Verification items for the finished model (mm, model axes). Face numbers are marked on the shaded views. Coordinates: 2 decimals unless noted, no trailing zeros. Order: outer loops, then holes, each group sorted by start corner. A loop starts at its lowest first (then second) coordinate and runs counter-clockwise, first axis right, second up. Notation, with made-up numbers: M 3,-6 L 38,-6 A19 ccw 38,7 Z; hole C -25.75,84 d6. An arc over 180 degrees is marked long. Return JSON: item names as keys, results as strings.
```python
from build123d import *

# Parameters (mm, degrees)
SKETCH1_W           = 400
SKETCH1_H           = 76.2
BOSS_EXTRUDE1_DEPTH = 50.8
SKETCH2_R           = 19
CUT_EXTRUDE1_DEPTH  = 76.2


with BuildPart() as part:
    # Sketch1 → Boss-Extrude1 (new body)
    with BuildSketch(Plane(origin=(0, 0, 0), x_dir=(1, 0, 0), z_dir=(0, 1, 0))):
        with Locations((200, 38.1)):
            Rectangle(SKETCH1_W, SKETCH1_H)
    extrude(amount=BOSS_EXTRUDE1_DEPTH)

    # Sketch2 → Cut-Extrude1 (cut)
    with BuildSketch(Plane.XY):
        with Locations((70, 25.4)):
            Circle(SKETCH2_R)
        with Locations((200, 25.4)):
            Circle(SKETCH2_R)
        with Locations((330, 25.4)):
            Circle(SKETCH2_R)
    extrude(amount=-CUT_EXTRUDE1_DEPTH, mode=Mode.SUBTRACT)


solid = part.part
```
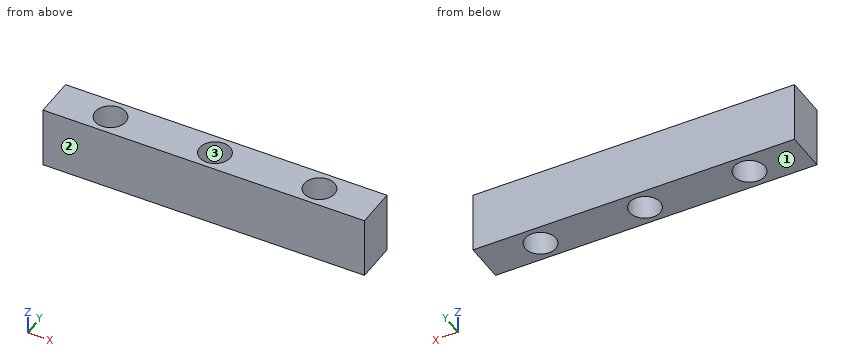
Q1. Cross-section at A-A, the plane y = 25.4. Record the boundary of the cut face in (x, z).
Values:
{"outline": "M 0,-76.2 L 51,-76.2 L 51,0 L 0,0 Z; M 89,-76.2 L 181,-76.2 L 181,0 L 89,0 Z; M 219,-76.2 L 311,-76.2 L 311,0 L 219,0 Z; M 349,-76.2 L 400,-76.2 L 400,0 L 349,0 Z"}
Q2. Cross-section at B-B, the plane x = 200. Record the boundary of the cut face in (y, z).
Values:
{"outline": "M 0,-76.2 L 6.4,-76.2 L 6.4,0 L 0,0 Z; M 44.4,-76.2 L 50.8,-76.2 L 50.8,0 L 44.4,0 Z"}
Q3. Cross-section at D-D, the plane x = 72. Record the boundary of the cut face in (y, z).
Values:
{"outline": "M 0,-76.2 L 6.51,-76.2 L 6.51,0 L 0,0 Z; M 44.29,-76.2 L 50.8,-76.2 L 50.8,0 L 44.29,0 Z"}
Q4. Go/stop test with a flat-tipped pin: pin 1 (23 mm diameter, centred on x = 70, y = 25.4, fed in from +Z). Record where the tip stops, or that it passes through.
Values:
{"pin 1": "through"}
Q5. Material ranges on line 1 along X through (y, z) = (24.5, -33); line 2 along Y through (x, z) = (200, -56); line 3 along X through (y, z) = (38.5, -53), recorded low to high.
Values:
{"line 1": "0 to 51.02, 88.98 to 181.02, 218.98 to 311.02, 348.98 to 400", "line 2": "0 to 6.4, 44.4 to 50.8", "line 3": "0 to 56.24, 83.76 to 186.24, 213.76 to 316.24, 343.76 to 400"}
Q6. Draft check along Y on the marked faces 1, 2 and 3. Enter one of: pulls with the +Y half, pulls with the -Y half, needs draft (parallel to the pull), parting line crosses it, or undercut.
Values:
{"face 1": "needs draft", "face 2": "pulls with the -Y half", "face 3": "undercut"}
Q7. Cross-section at C-C, the plane z = -63. Record the boundary of the cut face in (x, y), and give its area (3 significant figures).
Values:
{"outline": "M 0,0 L 400,0 L 400,50.8 L 0,50.8 Z; hole C 70,25.4 d38; hole C 200,25.4 d38; hole C 330,25.4 d38", "area": "16,900 mm^2"}
